Here's the drawing with two shaded views (mm, measured from the low corner). I have some questions. Round coordinates to 2 decimals unless told otherwise and drop trailing zeros. Order: outer loops, then holes, each group sorted by start corner. A loop starts at its lowest first (then second) coordinate and runs counter-clockwise, first axis right, second up. Notation, with made-up numbers: (22.25, -18.75) -> (32.25, -18.75) arc R11 ccw to (32.25, -12.75) -> close; hole circle Ø2 at (-8.5, 11.5). An arc over 180 degrees is marked (long way). Use a Markdown table: item, result. Add a question column.
Q1. If we section it at B-B on y = 24: List the corners of the cut face in (x, z) for me, plus the area to 4 significant figures.
Q2. If we section it at A-A on x = 132: List the corners of the cut face in (y, z) for me.
Q3. If we section it at C-C on z = 52.5: List the corners of the cut face in (x, y) for me, plus the area to 4 significant figures.
Q4. I'm going to push a flat-ended pin straight in: pin 1 Ø2.5 at (x, z) = (99, 177) entering from +Y. Where does the tip first touch, or does it pass through?
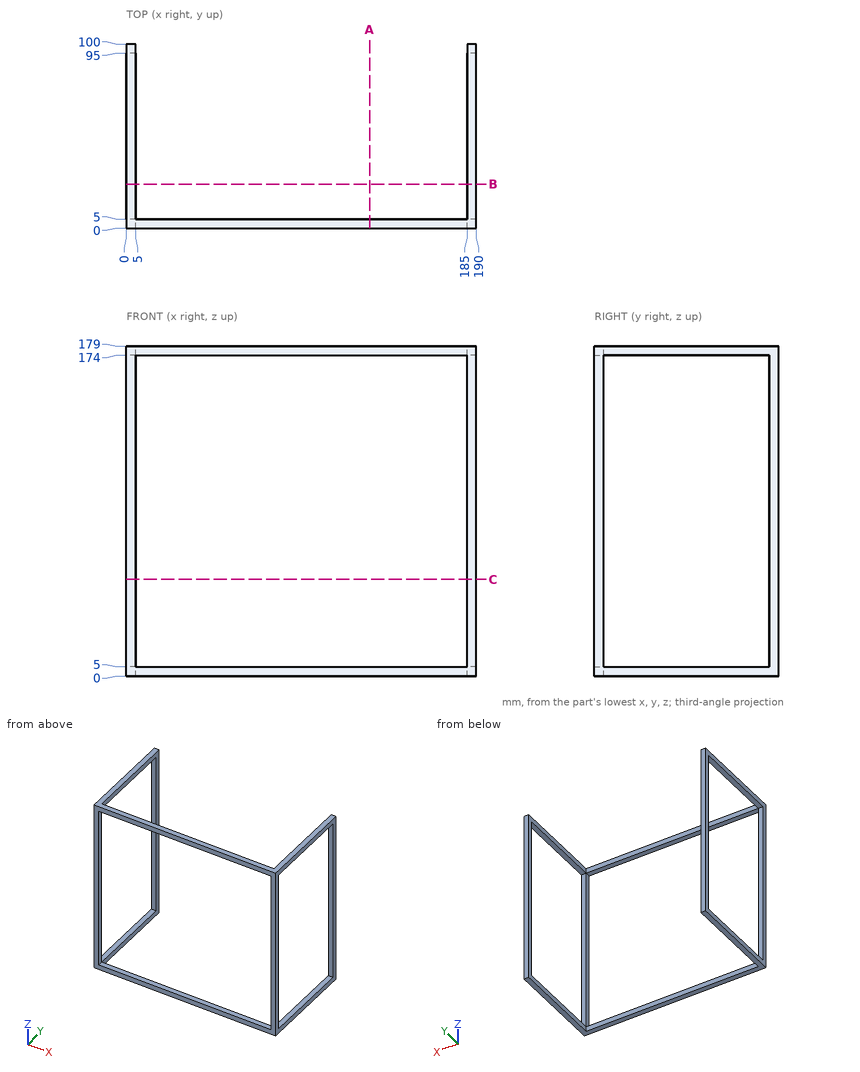
Answer below:
| question | item | result |
|---|---|---|
| 1 | outline | (0, 0) -> (5, 0) -> (5, 5) -> (0, 5) -> close; (0, 174) -> (5, 174) -> (5, 179) -> (0, 179) -> close; (185, 0) -> (190, 0) -> (190, 5) -> (185, 5) -> close; (185, 174) -> (190, 174) -> (190, 179) -> (185, 179) -> close |
| 1 | area | 100.0 mm² |
| 2 | outline | (0, 0) -> (5, 0) -> (5, 5) -> (0, 5) -> close; (0, 174) -> (5, 174) -> (5, 179) -> (0, 179) -> close |
| 3 | outline | (0, 0) -> (5, 0) -> (5, 5) -> (0, 5) -> close; (0, 95) -> (5, 95) -> (5, 100) -> (0, 100) -> close; (185, 0) -> (190, 0) -> (190, 5) -> (185, 5) -> close; (185, 95) -> (190, 95) -> (190, 100) -> (185, 100) -> close |
| 3 | area | 100.0 mm² |
| 4 | pin 1 | y = 5 |
